from build123d import *

# Parameters (mm, degrees)
SKETCH2_W           = 24
SKETCH2_H           = 45
BOSS_EXTRUDE1_DEPTH = 8
SKETCH5_W           = 24
SKETCH5_H           = 5
BOSS_EXTRUDE2_DEPTH = 15
SKETCH6_W           = 24
SKETCH6_H           = 5
BOSS_EXTRUDE3_DEPTH = 15
SKETCH7_R           = 1.5
CUT_EXTRUDE1_DEPTH  = 5
SKETCH8_R           = 1
CUT_EXTRUDE2_DEPTH  = 4


with BuildPart() as part:
    # Sketch2 → Boss-Extrude1 (new body)
    with BuildSketch(Plane(origin=(0, 0, 0), x_dir=(1, 0, 0), z_dir=(0, 1, 0))):
        with Locations((-7.196993829, 1.750308141)):
            Rectangle(SKETCH2_W, SKETCH2_H)
    extrude(amount=BOSS_EXTRUDE1_DEPTH)

    # Sketch5 → Boss-Extrude2 (add)
    with BuildSketch(Plane(origin=(0, 8, 0), x_dir=(1, 0, 0), z_dir=(0, 1, 0))):
        with Locations((-7.196993829, -18.249691859)):
            Rectangle(SKETCH5_W, SKETCH5_H)
    extrude(amount=BOSS_EXTRUDE2_DEPTH)

    # Sketch6 → Boss-Extrude3 (add)
    with BuildSketch(Plane.XZ):
        with Locations((-7.196993829, 18.249691859)):
            Rectangle(SKETCH6_W, SKETCH6_H)
    extrude(amount=BOSS_EXTRUDE3_DEPTH)

    # Sketch7 → Cut-Extrude1 (cut)
    with BuildSketch(Plane(origin=(0, 0, 15.749691859), x_dir=(-1, 0, 0), z_dir=(0, 0, -1))):
        with Locations((7.196993829, 15.5)):
            Circle(SKETCH7_R)
        with Locations((7.196993829, -7.5)):
            Circle(SKETCH7_R)
    extrude(amount=-CUT_EXTRUDE1_DEPTH, mode=Mode.SUBTRACT)

    # Sketch8 → Cut-Extrude2 (cut)
    with BuildSketch(Plane(origin=(0, 8, 0), x_dir=(1, 0, 0), z_dir=(0, 1, 0))):
        with Locations((-13.196993829, 21.250308141)):
            Circle(SKETCH8_R)
        with Locations((-1.196993829, 21.250308141)):
            Circle(SKETCH8_R)
    extrude(amount=-CUT_EXTRUDE2_DEPTH, mode=Mode.SUBTRACT)


solid = part.part
CAD build for the part. Positions are in the model's coordinates, mm. A direction names the side the tool comes from. Give positions to 0.01 mm unless a question says otherwise; leave off trailing zeros. Order: outer loops, then holes, each group sorted by start corner. A loop starts at its lowest first (then second) coordinate and runs counter-clockwise, first axis right, second up. Notation, with made-up numbers: (33.5, 49.25) - (82.5, 49.25) arc R23 cw to (82.5, 66.25) - close; hole circle Ø9 at (1, 25.25). An arc over 180 degrees is marked (long way). Answer in a Markdown table with one row per item.
1. Saw through at C-C, the plane z = 3. Give the cut face in (x, y).
Data:
| item | result |
|---|---|
| outline | (-19.2, 0) - (4.8, 0) - (4.8, 8) - (-19.2, 8) - close |
2. Pull direction Z, two halves, no side cores. Call faces 1 (the cylindrical face through (-1.414, 6.028, -20.274)), 2 (the flat face through (-7.4, -5.7, 15.75)), 3 (the flat face through (-7, 0, -5)): pulls with the +Z half, pulls with the -Z half, needs draft (parallel to the pull), parting line crosses it, or undercut.
Data:
| item | result |
|---|---|
| face 1 | undercut |
| face 2 | pulls with the -Z half |
| face 3 | needs draft |
3. Saw through at D-D, the plane y = -3.5. Give the cut face in (x, z).
Data:
| item | result |
|---|---|
| outline | (-19.2, 15.75) - (4.8, 15.75) - (4.8, 20.75) - (-19.2, 20.75) - close |
4. Tool access for faces 4 (the flat face through (4.803, 4, 5)), 5 (the cylindrical face through (-13.414, 6.028, -20.274)), 6 (the flat face through (-7, 8, -5)): list every direction of +Z, -Z, +X, -X, +Y, -Y with a clear straight run to the whole face (end or side of a thin tool).
Data:
| item | result |
|---|---|
| face 4 | +Z, -Z, +X, +Y, -Y |
| face 5 | +Y |
| face 6 | -Z, +X, -X, +Y |
5. Flat gauge pins, fed straight in: pin 1 (2.5 mm diameter, centred on x = -1.2, z = -21.25, fed in from -Y); pin 2 (1 mm diameter, centred on x = -1, z = -21, fed in from +Y); pin 3 (2.5 mm diameter, centred on x = -7.2, y = -7.5, fed in from +Z); pin 4 (2 mm diameter, centred on x = -13, z = -21.5, fed in from +Y). Where does each tip first touch, or does it go through?
Data:
| item | result |
|---|---|
| pin 1 | stops at y = 0 |
| pin 2 | stops at y = 4 |
| pin 3 | passes through |
| pin 4 | stops at y = 8 |
6. Probe probe 1 along Z at (x, y) = (-1.5, -12); probe 2 along Y at (x, z) = (4, -6); probe 3 along X at (y, z) = (15, 17). List the from-to ranges inside material, lowest first. Write a range as [from, to].
Data:
| item | result |
|---|---|
| probe 1 | z = [15.75, 20.75] |
| probe 2 | y = [0, 8] |
| probe 3 | x = [-19.2, -8.61], [-5.78, 4.8] |
7. Saw through at A-A, the plane y = -7.5. Give the cut face in (x, z).
Data:
| item | result |
|---|---|
| outline | (-19.2, 15.75) - (-8.7, 15.75) - (-8.7, 20.75) - (-19.2, 20.75) - close; (-5.7, 15.75) - (4.8, 15.75) - (4.8, 20.75) - (-5.7, 20.75) - close |
8. Saw through at B-B, the plane x = -3.5. Give the cut face in (y, z), plus the area to 3 significant figures.
Data:
| item | result |
|---|---|
| outline | (-15, 15.75) - (0, 15.75) - (0, -24.25) - (8, -24.25) - (8, 15.75) - (23, 15.75) - (23, 20.75) - (-15, 20.75) - close |
| area | 510 mm² |
